For this review, take the finished solid that the model builds, in its own axes (mm). Face numbers are marked on the shaded views. A direction names the side the tool comes from. Coordinates: 2 decimals unless noted, no trailing zeros. Loops run counter-clockwise (first coordinate to the right, second up) from the corner with the lowest first, then second, coordinate; pieces in that order, holes last. Notation, with made-up numbers: (2, 56.5) -> (59, 56.5) arc R15 ccw to (59, 83.5) -> close; hole circle Ø2 at (-20.5, 84.5). An arc over 180 degrees is marked (long way). One line per item, written item: value.
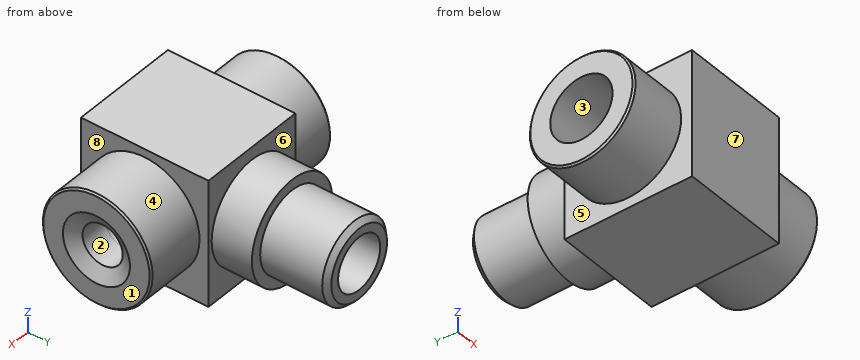
from build123d import *

# Parameters (mm, degrees)
SKETCH_1_W          = 32.4
SKETCH_1_H          = 38
EXTRUDE_1_DEPTH     = 37.5
SKETCH_4_R          = 15.75
EXTRUDE_2_DEPTH     = 17.5
SKETCH_5_R          = 9.3
CUT_EXTRUDE_1_DEPTH = 18
SKETCH_6_R          = 4
CUT_EXTRUDE_2_DEPTH = 2.4
SKETCH_7_R          = 2
CUT_EXTRUDE_3_DEPTH = 18.6
SKETCH_8_R          = 16.35
EXTRUDE_3_DEPTH     = 18
SKETCH_9_R          = 6
CUT_EXTRUDE_4_DEPTH = 12.5
CHAMFER_1_SIZE      = 4
CHAMFER_1_SIZE2     = 2.309401077
SKETCH_10_R         = 2.5
CUT_EXTRUDE_5_DEPTH = 21.7
FILLET_1_R          = 2
SKETCH_11_R         = 15
EXTRUDE_4_DEPTH     = 12
SKETCH_12_R         = 11.9
EXTRUDE_5_DEPTH     = 20
SKETCH_13_R         = 7.85
CUT_EXTRUDE_6_DEPTH = 17
SKETCH_14_R         = 4.5
CUT_EXTRUDE_7_DEPTH = 42
CHAMFER_2_SIZE      = 1.5
CHAMFER_4_SIZE      = 0.5
CHAMFER_5_SIZE      = 0.5
SKETCH_15_R         = 3.5
CUT_EXTRUDE_8_DEPTH = 6
CHAMFER_6_SIZE      = 5
CHAMFER_6_SIZE2     = 2.500539856


with BuildPart() as part:
    # Эскиз1 → Бобышка-Вытянуть1 (new body)
    with BuildSketch(Plane.XY):
        with Locations((16.2, 19)):
            Rectangle(SKETCH_1_W, SKETCH_1_H)
    extrude(amount=EXTRUDE_1_DEPTH)

    # Эскиз4 → Бобышка-Вытянуть2 (add)
    with BuildSketch(Plane.ZY):
        with Locations((18.75, 19)):
            Circle(SKETCH_4_R)
    extrude(amount=EXTRUDE_2_DEPTH)

    # Эскиз5 → Вырез-Вытянуть1 (cut)
    with BuildSketch(Plane.ZY.offset(17.5)):
        with Locations((18.75, 19)):
            Circle(SKETCH_5_R)
    extrude(amount=-CUT_EXTRUDE_1_DEPTH, mode=Mode.SUBTRACT)

    # Эскиз6 → Вырез-Вытянуть2 (cut)
    with BuildSketch(Plane.ZY.offset(-0.5)):
        with Locations((18.75, 19)):
            Circle(SKETCH_6_R)
    extrude(amount=-CUT_EXTRUDE_2_DEPTH, mode=Mode.SUBTRACT)

    # Эскиз7 → Вырез-Вытянуть3 (cut)
    with BuildSketch(Plane.ZY.offset(-0.5)):
        with Locations((18.75, 15)):
            Circle(SKETCH_7_R)
    extrude(amount=-CUT_EXTRUDE_3_DEPTH, mode=Mode.SUBTRACT)

    # Эскиз8 → Бобышка-Вытянуть3 (add)
    with BuildSketch(Plane(origin=(32.4, 0, 0), x_dir=(0, 0, -1), z_dir=(1, 0, 0))):
        with Locations((-18.75, 19)):
            Circle(SKETCH_8_R)
    extrude(amount=EXTRUDE_3_DEPTH)

    # Эскиз9 → Вырез-Вытянуть4 (cut)
    with BuildSketch(Plane(origin=(50.4, 0, 0), x_dir=(0, 0, -1), z_dir=(1, 0, 0))):
        with Locations((-18.75, 19)):
            Circle(SKETCH_9_R)
    extrude(amount=-CUT_EXTRUDE_4_DEPTH, mode=Mode.SUBTRACT)

    # Фаска1
    chamfer_1_edges = [part.edges().sort_by_distance(p)[0] for p in [
        (50.4, 19, 24.75),
    ]]
    chamfer_1_side = [part.faces().sort_by_distance(p)[0] for p in [
        (50.4, 19, 34.637552165),
    ]]
    chamfer(chamfer_1_edges, length=CHAMFER_1_SIZE, length2=CHAMFER_1_SIZE2, reference=chamfer_1_side[0])

    # Эскиз10 → Вырез-Вытянуть5 (cut)
    with BuildSketch(Plane(origin=(37.9, 0, 0), x_dir=(0, 0, -1), z_dir=(1, 0, 0))):
        with Locations((-18.75, 19)):
            Circle(SKETCH_10_R)
    extrude(amount=-CUT_EXTRUDE_5_DEPTH, mode=Mode.SUBTRACT)

    # Скругление1
    fillet_1_edges = [part.edges().sort_by_distance(p)[0] for p in [
        (37.9, 19, 24.75),
    ]]
    fillet(fillet_1_edges, radius=FILLET_1_R)

    # Эскиз11 → Бобышка-Вытянуть4 (add)
    with BuildSketch(Plane(origin=(0, 38, 0), x_dir=(1, 0, 0), z_dir=(0, 1, 0))):
        with Locations((16.2, -18.75)):
            Circle(SKETCH_11_R)
    extrude(amount=EXTRUDE_4_DEPTH)

    # Эскиз12 → Бобышка-Вытянуть5 (add)
    with BuildSketch(Plane(origin=(0, 50, 0), x_dir=(1, 0, 0), z_dir=(0, 1, 0))):
        with Locations((16.2, -18.75)):
            Circle(SKETCH_12_R)
    extrude(amount=EXTRUDE_5_DEPTH)

    # Эскиз13 → Вырез-Вытянуть6 (cut)
    with BuildSketch(Plane(origin=(0, 70, 0), x_dir=(1, 0, 0), z_dir=(0, 1, 0))):
        with Locations((16.2, -18.75)):
            Circle(SKETCH_13_R)
    extrude(amount=-CUT_EXTRUDE_6_DEPTH, mode=Mode.SUBTRACT)

    # Эскиз14 → Вырез-Вытянуть7 (cut)
    with BuildSketch(Plane(origin=(0, 53, 0), x_dir=(1, 0, 0), z_dir=(0, 1, 0))):
        with Locations((16.2, -18.75)):
            Circle(SKETCH_14_R)
    extrude(amount=-CUT_EXTRUDE_7_DEPTH, mode=Mode.SUBTRACT)

    # Фаска2
    chamfer_2_edges = [part.edges().sort_by_distance(p)[0] for p in [
        (4.3, 70, 18.75),
    ]]
    chamfer(chamfer_2_edges, length=CHAMFER_2_SIZE)

    # Фаска4
    chamfer_4_edges = [part.edges().sort_by_distance(p)[0] for p in [
        (-17.5, 19, 3),
    ]]
    chamfer(chamfer_4_edges, length=CHAMFER_4_SIZE)

    # Фаска5
    chamfer_5_edges = [part.edges().sort_by_distance(p)[0] for p in [
        (50.4, 19, 35.1),
    ]]
    chamfer(chamfer_5_edges, length=CHAMFER_5_SIZE)

    # Эскиз15 → Вырез-Вытянуть8 (cut)
    with BuildSketch(Plane(origin=(0, 11, 0), x_dir=(1, 0, 0), z_dir=(0, 1, 0))):
        with Locations((16.2, -18.75)):
            Circle(SKETCH_15_R)
    extrude(amount=-CUT_EXTRUDE_8_DEPTH, mode=Mode.SUBTRACT)

    # Фаска6
    chamfer_6_edges = [part.edges().sort_by_distance(p)[0] for p in [
        (12.7, 5, 18.75),
    ]]
    chamfer_6_side = [part.faces().sort_by_distance(p)[0] for p in [
        (12.7, 8, 18.75),
    ]]
    chamfer(chamfer_6_edges, length=CHAMFER_6_SIZE, length2=CHAMFER_6_SIZE2, reference=chamfer_6_side[0])


solid = part.part
1. The part is to be moulded in two halves that separate along Z. For the marked faces 1, 2, 3 and 4, say which applies: pulls with the +Z half, pulls with the -Z half, needs draft (parallel to the pull), parting line crosses it, or undercut.
Return value:
face 1: needs draft
face 2: undercut
face 3: undercut
face 4: parting line crosses it
2. For the marked faces 5, 6, 7 and 8, list the 3-axis set-ups (+Z, -Z, +X, -X, +Y, -Y) from which the entire face can be reached by the end or side of a thin tool; tool diameter is ignored.
Return value:
face 5: -X
face 6: +Y
face 7: +Z, -Z, +X, -X, -Y
face 8: +X
3. Take a section at D-D, the plane x = 41.5. Give the boundary of the cut face in (y, z), and give its area (3 significant figures).
Return value:
outline: circle Ø32.7 at (19, 18.75); hole circle Ø12 at (19, 18.75)
area: 727 mm2
4. To check wall thickness, follow probe 1 along Z at (x, y) = (1.45, 19); probe 2 along Z at (x, y) = (9.5, 15); probe 3 along X at (y, z) = (40.5, 18.75). State the ranges of each line that lie inside material, in increasing order. Write a range as from..to.
Return value:
probe 1: z = 0..14.75, 22.75..37.5
probe 2: z = 0..16.75, 20.75..37.5
probe 3: x = 1.2..11.7, 20.7..31.2
5. Take a section at C-C, the plane z = 18.75. Give the number of separate pieces and of enclosed holes in the cut face, and give its area (3 significant figures).
Return value:
separate pieces: 3
enclosed holes: 0
area: 1,890 mm2
6. Take a section at B-B, the plane y = 45. Give the boundary of the cut face in (x, z).
Return value:
outline: circle Ø30 at (16.2, 18.75); hole circle Ø9 at (16.2, 18.75)
7. Insertion check: pin 1 Ø9 at (y, z) = (19.5, 18) entering from +X; pin 2 Ø11 at (y, z) = (19, 18.75) entering from +X; pin 3 Ø10.5 at (y, z) = (19, 18.75) entering from -X. Each pin has a flat end and moves straight along its axis. Give the tip position at first contact, or say it passes through.
Return value:
pin 1: stops at x = 38.47
pin 2: stops at x = 38.58
pin 3: stops at x = 0.5
8. Take a section at A-A, the plane x = 16.2. Give the boundary of the cut face in (y, z).
Return value:
outline: (0, 0) -> (38, 0) -> (38, 3.75) -> (50, 3.75) -> (50, 6.85) -> (68.5, 6.85) -> (70, 8.35) -> (70, 10.9) -> (53, 10.9) -> (53, 14.25) -> (11, 14.25) -> (11, 15.25) -> (10, 15.25) -> (5, 17.75) -> (5, 19.75) -> (10, 22.25) -> (11, 22.25) -> (11, 23.25) -> (53, 23.25) -> (53, 26.6) -> (70, 26.6) -> (70, 29.15) -> (68.5, 30.65) -> (50, 30.65) -> (50, 33.75) -> (38, 33.75) -> (38, 37.5) -> (0, 37.5) -> close
